Here's how the part is built. I have some questions about the finished solid (model axes, mm). Face numbers are marked on the shaded views. A direction names the side the tool comes from. Round coordinates to 2 decimals unless told otherwise and drop trailing zeros. Write each loop counter-clockwise with the first axis right and the second up, starting at its lowest first coordinate (ties: lowest second). Pieces come first, ordered by that corner, then holes. Notation, with made-up numbers: M 40,22.25 L 46,22.25 A15 ccw 46,26.25 Z; hole C -11,24 d8. An arc over 180 degrees is marked long. Use one line per item in the form item = value. Start each with the question number.
Q1. I want a section at A-A on x = 0. List the corners of the cut face in (y, z) for me.
Q2. For the marked faces 1 and 2, which set-ups out of +Z, -Z, +X, -X, +Y, -Y let a thin tool reach every point of the face, with its end or its side?
Q3. I want a section at D-D on y = -11.25. List the corners of the cut face in (x, z) for me.
Q4. I want a section at B-B on z = 2.75. List the corners of the cut face in (x, y) for me, and give its area (3 significant figures).
Q5. I want a section at C-C on z = 8. List the corners of the cut face in (x, y) for me.
Q6. I need wall thicknesses on line 1 along X through (y, z) = (-5.5, 8); line 2 along X through (y, z) = (-4.5, 4.5); line 3 along X through (y, z) = (-7.5, 2.1). Which ranges of each line are inside material? Lowest first, please. Write a range as from..to.
Q7. We'd pull the mould along Z, two halves only. Please class the marked faces 3, 4 and 5: +Z half, -Z half, draft (parallel to the pull), parting line (faces both ways), or undercut.
Q8. I'm going to push flat-ended pins straight in: pin 1 Ø9 at (x, y) = (0, -7.5) entering from -Z; pin 2 Ø6 at (x, z) = (4, 5.5) entering from +Y; pin 3 Ø1.5 at (x, y) = (-4, -7.5) entering from -Z. Where does each tip first touch, or does it pass through?
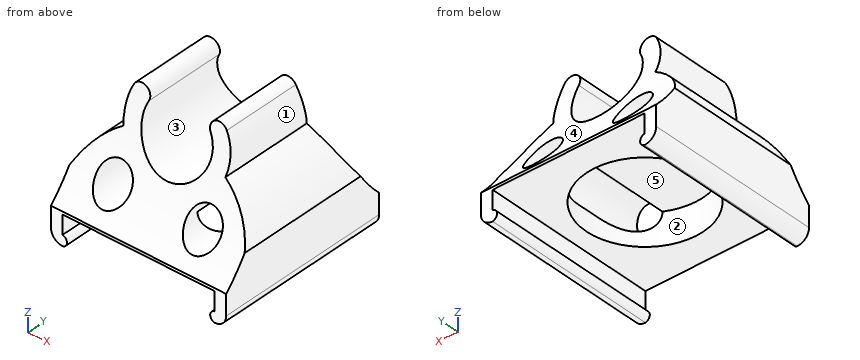
```python
from build123d import *

# Parameters (mm, degrees)
F0_R          = 1.5
F1_DEPTH      = 15
F2_R          = 14.550115737
F3_DEPTH      = 25
F3_DEPTH_BACK = 25
F4_R          = 5
F5_DEPTH      = 3.5


# Not quite as in the source:
# - ends of sketch curves that miss each other by under 0.0002 mm in the source are joined


with BuildPart() as f1:
    # F0 (on Front) → F1 (new body)
    with BuildSketch(Plane.XZ):
        with BuildLine():
            Line((-6.5, -0.8), (-6.5, 0.8))
            Line((-6.5, 0.8), (6.5, 0.8))
            Line((6.5, 0.8), (6.5, -0.8))
            ThreePointArc((6.5, -0.8), (6.1264578545, -1.2499931592), (6.4999470351, -1.7000302796))
            ThreePointArc((6.4999470351, -1.7000302796), (7.2070390333, -1.4071599085), (7.4999451737, -0.7000767547))
            Line((7.4999451737, -0.7000767547), (7.5000913757, 3.3000402053))
            ThreePointArc((7.5000913757, 3.3000402053), (6.2070011857, 5.3492777345), (4.3711160801, 6.93072725))
            ThreePointArc((4.3711160801, 6.93072725), (4.4644607322, 8.5644381014), (3.967454999, 10.1235114388))
            ThreePointArc((3.967454999, 10.1235114388), (2.952293926, 10.4308353655), (2.6449699993, 9.4156742925))
            ThreePointArc((2.6449699993, 9.4156742925), (0, 5), (-2.6449699993, 9.4156742925))
            ThreePointArc((-2.6449699993, 9.4156742925), (-2.952293926, 10.4308353655), (-3.967454999, 10.1235114388))
            ThreePointArc((-3.967454999, 10.1235114388), (-4.4644607322, 8.5644381014), (-4.3711160801, 6.93072725))
            ThreePointArc((-4.3711160801, 6.93072725), (-6.2070011857, 5.3492777345), (-7.5000913757, 3.3000402053))
            Line((-7.5000913757, 3.3000402053), (-7.4999451737, -0.7000767547))
            ThreePointArc((-7.4999451737, -0.7000767547), (-7.2070390333, -1.4071599085), (-6.4999451744, -1.7000402053))
            ThreePointArc((-6.4999451744, -1.7000402053), (-6.1264578541, -1.2500021402), (-6.5, -0.8))
        make_face()
        with Locations((-3.848537337, 3.4744446166)):
            Circle(F0_R, mode=Mode.SUBTRACT)
        with Locations((3.848537337, 3.4744446166)):
            Circle(F0_R, mode=Mode.SUBTRACT)
    extrude(amount=F1_DEPTH)

    # F2 (on Right) → F3 (cut, two sides)
    with BuildSketch(Plane.YZ) as f3_sk:
        with Locations((-25.4004554451, 11.2085361034)):
            Circle(F2_R)
        with Locations((10.4004554451, 11.2085361034)):
            Circle(F2_R)
    extrude(amount=-F3_DEPTH, mode=Mode.SUBTRACT)
    extrude(f3_sk.sketch, amount=F3_DEPTH_BACK, mode=Mode.SUBTRACT)

    # F4 (on Top) → F5 (cut)
    with BuildSketch(Plane.XY):
        with Locations((0, -7.5)):
            Circle(F4_R)
    extrude(amount=F5_DEPTH, mode=Mode.SUBTRACT)


solid = f1.part
```
Reported:
q1.outline = M -15,0.8 L -12.5,0.8 L -12.5,3.5 L -2.5,3.5 L -2.5,0.8 L 0,0.8 L 0,1.03 A14.55 cw -2.76,5 L -12.24,5 A14.55 cw -15,1.03 Z
q2.face_1 = +X, +Y, -Y
q2.face_2 = -Z
q3.outline = M -7.5,-0.7 A1 ccw -6.5,-1.7 A0.46 ccw -6.5,-0.8 L -6.5,0.8 L -3.31,0.8 L -3.31,2.08 A1.5 cw long -2.35,3.5 L 2.35,3.5 A1.5 cw long 3.31,2.08 L 3.31,0.8 L 6.5,0.8 L 6.5,-0.8 A0.46 ccw 6.5,-1.7 A1 ccw 7.5,-0.7 L 7.5,3.3 A8.19 ccw 4.37,6.93 A4.5 ccw 4.5,7.82 L 2.99,7.82 A3 cw -2.99,7.82 L -4.5,7.82 A4.5 ccw -4.37,6.93 A8.19 ccw -7.5,3.3 Z
q4.outline = M -7.5,-13.56 L -5.16,-13.56 L -5.16,-1.44 L -7.5,-1.44 Z; M -2.54,-13.56 L 2.54,-13.56 L 2.54,-11.81 A5 cw -2.54,-11.81 Z; M -2.54,-3.19 A5 cw 2.54,-3.19 L 2.54,-1.44 L -2.54,-1.44 Z; M 5.16,-13.56 L 7.5,-13.56 L 7.5,-1.44 L 5.16,-1.44 Z
q4.area = 69.7 mm^2
q5.outline = M -4.5,-11.21 L -3,-11.21 L -3,-3.79 L -4.5,-3.79 Z; M 3,-11.21 L 4.5,-11.21 L 4.5,-3.79 L 3,-3.79 Z
q6.line_1 = -4.5..-3, 3..4.5
q6.line_2 = -6.85..-4.94, -2.75..2.75, 4.94..6.85
q6.line_3 = -7.5..-5, 5..7.5
q7.face_3 = undercut
q7.face_4 = +Z half
q7.face_5 = -Z half
q8.pin_1 = 3.5
q8.pin_2 = -1.42
q8.pin_3 = 4.67
